Check sheet for the modelled part. Datum: model origin and axes. Units: mm. Give positions to 0.01 mm unless a question says otherwise; leave off trailing zeros. Write each loop counter-clockwise with the first axis right and the second up, starting at its lowest first coordinate (ties: lowest second). Pieces come first, ordered by that corner, then holes. Notation, with made-up numbers: (43, 1) -> (94, 1) arc R26 ccw to (94, 26) -> close; hole circle Ø1 at (-34.5, 60). An arc over 180 degrees is marked (long way). Return JSON: item names as keys, results as strings.
Autodesk Inventor part; units mm, degrees
ref_plane "YZ Plane" through (0, 0, 0) normal (1, 0, 0) x (0, 1, 0)
ref_plane "XZ Plane" through (0, 0, 0) normal (0, 1, 0) x (-1, 0, 0)
ref_plane "XY Plane" through (0, 0, 0) normal (0, 0, 1) x (1, 0, 0)
sketch "Sketch1" plane through (0, 0, 0) normal (0, 1, 0) x (-1, 0, 0)
  line L0 (-3.175, -3.175) -> (3.175, -3.175)
  line L1 (3.175, -3.175) -> (3.175, 3.175)
  line L2 (3.175, 3.175) -> (-3.175, 3.175)
  line L3 (-3.175, 3.175) -> (-3.175, -3.175)
  line L4 (-3.175, -3.175) -> (3.175, 3.175) construction
  line L5 (3.175, -3.175) -> (-3.175, 3.175) construction
  point P0 (0, 0)
  dimension "d0" = 6.35
  dimension "d1" = 6.35
extrude "Extrusion1" add sketch "Sketch1" along normal blind 88.9
sketch "Sketch2" plane through (-3.175, 0, 3.175) normal (0, 0, 1) x (1, 0, 0)
  circle A0 centre (3.175, 6.35) radius 2.159
  line L0 (0, 0) -> (6.35, 0)
  circle A1 centre (3.175, 82.55) radius 2.159
  line L1 (0, 88.9) -> (6.35, 88.9)
  point P0 (3.175, 0)
  dimension "d4" = 4.318
  dimension "d5" = 6.35
  dimension "d6" = 4.318
  dimension "d7" = 6.35
extrude "Extrusion2" cut sketch "Sketch2" against normal blind 88.9
fillet "Fillet1" radius 1.5875 4 edges at (3.175, 44.45, -3.175) (-3.175, 44.45, -3.175) (3.175, 44.45, 3.175) (-3.175, 44.45, 3.175)
fillet "Fillet2" radius 0.7937 16 edges at (2.71, 88.9, -2.71) (0, 88.9, -3.175) (-2.71, 88.9, -2.71) (-3.175, 88.9, 0) (-2.71, 88.9, 2.71) (0, 88.9, 3.175) (2.71, 88.9, 2.71) (3.175, 88.9, 0) (0, 0, -3.175) (-2.71, 0, -2.71) (-3.175, 0, 0) (-2.71, 0, 2.71) (0, 0, 3.175) (2.71, 0, 2.71) (3.175, 0, 0) (2.71, 0, -2.71)
properties part number "45 stop" material "Stainless Steel"
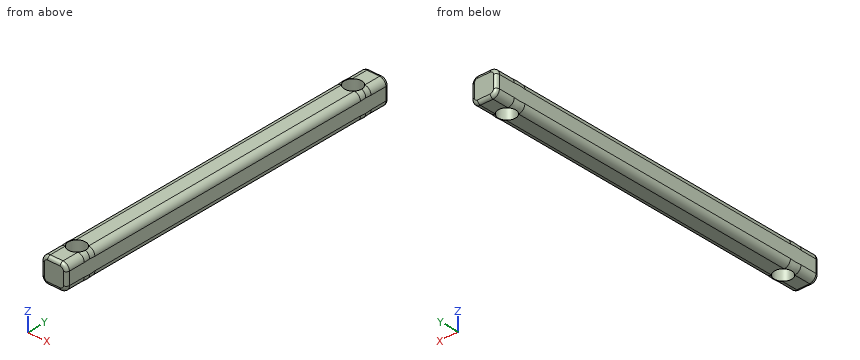
(1) Cross-section at A-A on x = 0. Enter the section's corners in (y, z) (3 decimals), then the cut area to 3 significant figures.
Reply:
{"outline": "(0, -2.381) arc R0.794 ccw to (0.794, -3.175) -> (4.191, -3.175) -> (4.191, 3.175) -> (0.794, 3.175) arc R0.794 ccw to (0, 2.381) -> close; (8.509, -3.175) -> (80.391, -3.175) -> (80.391, 3.175) -> (8.509, 3.175) -> close; (84.709, -3.175) -> (88.106, -3.175) arc R0.794 ccw to (88.9, -2.381) -> (88.9, 2.381) arc R0.794 ccw to (88.106, 3.175) -> (84.709, 3.175) -> close", "area": "509 mm^2"}
(2) Thickness scan on L1, parallel to X at y = 6.35, z = 1.25 (3 decimals); L2, parallel to Y at x = 1.25, z = 1; L3, parallel to Y at x = 1.5, z = 0. Record the ranges inside material, lowest first.
Reply:
{"L1": "-3.175 to -2.159, 2.159 to 3.175", "L2": "0 to 4.59, 8.11 to 80.79, 84.31 to 88.9", "L3": "0 to 4.8, 7.9 to 81, 84.1 to 88.9"}
(3) Cross-section at C-C on y = 47. Enter the section's corners in (x, z) (1 decimal), then the cut area to 3 significant figures.
Reply:
{"outline": "(-3.2, -1.6) arc R1.6 ccw to (-1.6, -3.2) -> (1.6, -3.2) arc R1.6 ccw to (3.2, -1.6) -> (3.2, 1.6) arc R1.6 ccw to (1.6, 3.2) -> (-1.6, 3.2) arc R1.6 ccw to (-3.2, 1.6) -> close", "area": "38.2 mm^2"}
(4) Depth check by flat-ended pin: pin 1 Ø3.5 at (x, y) = (0, 82.55) entering from +Z. Enter the tip coordinate at first touch or a pass-through.
Reply:
{"pin 1": "through"}
(5) Cross-section at B-B on z = 0.75. Enter the section's corners in (x, y) (3 decimals).
Reply:
{"outline": "(-3.175, 0.794) arc R0.794 ccw to (-2.381, 0) -> (2.381, 0) arc R0.794 ccw to (3.175, 0.794) -> (3.175, 88.106) arc R0.794 ccw to (2.381, 88.9) -> (-2.381, 88.9) arc R0.794 ccw to (-3.175, 88.106) -> close; hole circle Ø4.318 at (0, 6.35); hole circle Ø4.318 at (0, 82.55)"}
